Here's how the part is built. I have some questions about the finished solid (model axes, mm). A direction names the side the tool comes from. Round coordinates to 2 decimals unless told otherwise and drop trailing zeros. Order: outer loops, then holes, each group sorted by start corner. A loop starts at its lowest first (then second) coordinate and runs counter-clockwise, first axis right, second up.
```python
from build123d import *

# Parameters (mm, degrees)
F0_R      = 19.8409660839
F1_DEPTH  = 38.1
F3_W      = 40.1443894953
F3_H      = 12.2663397342
F4_DEPTH  = 64.262
F5_W      = 40.7019536942
F5_H      = 9.4785336405
F6_DEPTH  = 64.262
F7_D      = 12.7
F9_DEPTH  = 12.192
F11_DEPTH = 9.398


with BuildPart() as f1:
    # F0 (on Front) → F1 (new body, symmetric)
    with BuildSketch(Plane.XZ):
        Circle(F0_R)
    extrude(amount=F1_DEPTH, both=True)

    # F3 (on Top) → F4 (join)
    with BuildSketch(Plane.XY):
        with Locations((-0.1393901184, -31.7809758708)):
            Rectangle(F3_W, F3_H)
    extrude(amount=F4_DEPTH)

    # F5 (on Top) → F6 (join)
    with BuildSketch(Plane.XY):
        with Locations((-0.1393901184, 33.1748789176)):
            Rectangle(F5_W, F5_H)
    extrude(amount=F6_DEPTH)

    # F7 (through all)
    with Locations(Plane(origin=(0, 38.1, 0), x_dir=(-1, 0, 0), z_dir=(0, 1, 0))):
        with Locations((0, 0)):
            Hole(F7_D / 2)

    # F8 (on face) → F9 (join)
    with BuildSketch(Plane(origin=(0, -25.6478060037, 0), x_dir=(-1, 0, 0), z_dir=(0, 1, 0))):
        with BuildLine():
            Line((-19.566863193, 64.262), (19.566863193, 64.262))
            ThreePointArc((19.566863193, 64.262), (0, 83.828863193), (-19.566863193, 64.262))
        make_face()
    extrude(amount=-F9_DEPTH)

    # F10 (on face) → F11 (join)
    with BuildSketch(Plane(origin=(0, 37.9141457379, 0), x_dir=(-1, 0, 0), z_dir=(0, 1, 0))):
        with BuildLine():
            Line((-19.8116342985, 64.262), (20.0904145353, 64.262))
            ThreePointArc((20.0904145353, 64.262), (0.1393901184, 84.2130244169), (-19.8116342985, 64.262))
        make_face()
    extrude(amount=-F11_DEPTH)


solid = f1.part
```
1) I need wall thicknesses on line 1 (Y direction, x = 17, z = 69); line 2 (Z direction, x = 0, y = 9); line 3 (Y direction, x = -2, z = 49.5). Which ranges of each line are inside material? Lowest first, please.
2) For faces 4 (the flat face through (-5, -38.1, 5)), 5 (the flat face through (-20.212, -32, 32)), 6 (the flat face through (0, -37.84, 72)), 7 (the flat face through (0, 28.516, 72)), 8 (the cylindrical face through (9.16, -0.53, -17.6)), which set-ups out of +Z, -Z, +X, -X, +Y, -Y let a thin tool reach every point of the face, with its end or its side?
3) We'd pull the mould along Z, two halves only. Please class faces 1 (the cylindrical face through (-0.43, -31.658, 83.824)), 2 (the flat face through (19.933, -32, 32)), 3 (the cylindrical face through (-1.38, -0.53, -6.2)): +Z half, -Z half, draft (parallel to the pull), parting line (faces both ways), or undercut.
4) If we section it at C-C (x = 0): Write out the boundary of the cut face in (y, z).
5) I'm going to push flat-ended pins straight in: pin 1 (1 mm diameter, centred on x = 3.5, z = 21.5, fed in from +Y); pin 2 (10 mm diameter, centred on x = -7.5, y = 21.5, fed in from +Z); pin 3 (13.5 mm diameter, centred on y = -33.5, z = 44.5, fed in from +X); pin 4 (10 mm diameter, centred on x = 0, z = 0, fed in from +Y). Where does each tip first touch, or does it pass through?
6) If we section it at A-A (y = 33): Write out the boundary of the cut face in (x, z), plus the area to 3 significant figures.
7) If we section it at B-B (z = 29): Write out the boundary of the cut face in (x, y).
8) If we section it at D-D (x = 12): Write out the boundary of the cut face in (y, z).
Solutions:
1. line 1: y = -37.84 to -25.65, 28.52 to 37.91
1. line 2: z = -19.84 to -6.35, 6.35 to 19.84
1. line 3: y = -37.91 to -25.65, 28.44 to 37.91
2. face 4: +Z, -Z, +X, -X, -Y
2. face 5: +Z, -Z, -X, -Y
2. face 6: +Z, +X, -X, -Y
2. face 7: +Z, +X, -X
2. face 8: none
3. face 1: +Z half
3. face 2: draft
3. face 3: undercut
4. outline: (-38.1, -19.84) - (38.1, -19.84) - (38.1, -6.35) - (-38.1, -6.35) - close; (-38.1, 6.35) - (38.1, 6.35) - (38.1, 19.84) - (37.91, 19.84) - (37.91, 84.21) - (28.52, 84.21) - (28.52, 64.26) - (28.44, 64.26) - (28.44, 19.84) - (-25.65, 19.84) - (-25.65, 83.83) - (-37.84, 83.83) - (-37.84, 64.26) - (-37.91, 64.26) - (-37.91, 19.84) - (-38.1, 19.84) - close
5. pin 1: stops at y = 37.91
5. pin 2: stops at z = 19.68
5. pin 3: stops at x = 19.93
5. pin 4: passes through
6. outline: (-20.49, 0) - (-19.84, 0) arc R19.84 ccw to (19.84, 0) - (20.21, 0) - (20.21, 64.26) - (19.81, 64.26) arc R19.95 ccw to (-20.09, 64.26) - (-20.49, 64.26) - close; hole circle Ø12.7 at (0, 0)
6. area: 3,730 mm2
7. outline: (-20.49, 28.44) - (20.21, 28.44) - (20.21, 37.91) - (-20.49, 37.91) - close; (-20.21, -37.91) - (19.93, -37.91) - (19.93, -25.65) - (-20.21, -25.65) - close
8. outline: (-38.1, -15.8) - (38.1, -15.8) - (38.1, 15.8) - (37.91, 15.8) - (37.91, 80.09) - (28.52, 80.09) - (28.52, 64.26) - (28.44, 64.26) - (28.44, 15.8) - (-25.65, 15.8) - (-25.65, 79.72) - (-37.84, 79.72) - (-37.84, 64.26) - (-37.91, 64.26) - (-37.91, 15.8) - (-38.1, 15.8) - close
